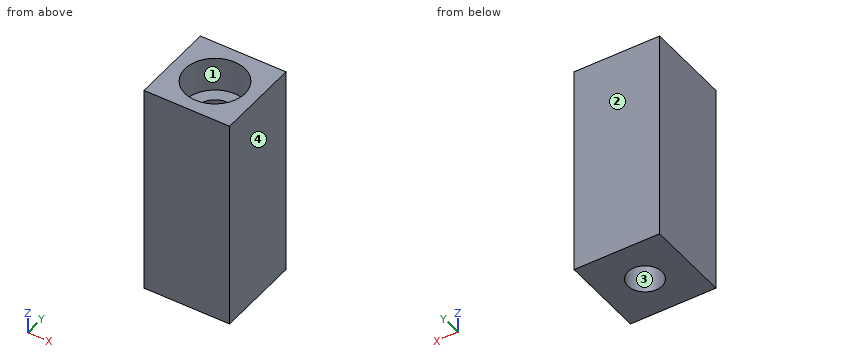
Autodesk Inventor part; units mm, degrees
ref_plane "YZ Plane" through (0, 0, 0) normal (1, 0, 0) x (0, 1, 0)
ref_plane "XZ Plane" through (0, 0, 0) normal (0, 1, 0) x (-1, 0, 0)
ref_plane "XY Plane" through (0, 0, 0) normal (0, 0, 1) x (1, 0, 0)
sketch "Sketch1" plane through (0, 0, 0) normal (0, 0, 1) x (1, 0, 0)
  line L0 (-5, -5) -> (5, -5)
  line L1 (5, -5) -> (5, 5)
  line L2 (5, 5) -> (-5, 5)
  line L3 (-5, 5) -> (-5, -5)
  line L4 (-5, -5) -> (5, 5) construction
  line L5 (5, -5) -> (-5, 5) construction
  point P0 (0, 0)
  dimension "length" = 10
  dimension "d1" = 10
extrude "Extrusion1" add sketch "Sketch1" along normal blind 25
sketch "Sketch2" plane through (0, 0, 25) normal (0, 0, 1) x (1, 0, 0)
  circle A0 centre (0, 0) radius 3.5
  dimension "diameter" = 7
extrude "Extrusion2" cut sketch "Sketch2" against normal blind 4
sketch "Sketch3" plane through (0, 0, 21) normal (0, 0, 1) x (1, 0, 0)
  circle A0 centre (0, 0) radius 2
  dimension "d9" = 4
extrude "Extrusion3" cut sketch "Sketch3" against normal blind 21
thread "Thread3"
equation "\"d1\" = length"
equation "\"d14\" = length"
properties part number "m4x0.7 25mm long"
For this review, take the finished solid that the model builds, in its own axes (mm). Face numbers are marked on the shaded views. Give positions to 0.01 mm unless a question says otherwise; leave off trailing zeros. Write each loop counter-clockwise with the first axis right and the second up, starting at its lowest first coordinate (ties: lowest second). Pieces come first, ordered by that corner, then holes. Notation, with made-up numbers: M 86,86.25 L 91,86.25 A18 cw 91,115.25 Z; hole C -31,15.5 d8. An arc over 180 degrees is marked long. One line per item, written item: value.
1) Take a section at C-C, the plane z = 8.25. Write out the cut boundary in (x, y).
Results are:
outline: M -5,-5 L 5,-5 L 5,5 L -5,5 Z; hole C 0,0 d4
2) Take a section at A-A, the plane y = 0. Write out the cut boundary in (x, z).
Results are:
outline: M -5,0 L -2,0 L -2,21 L -3.5,21 L -3.5,25 L -5,25 Z; M 2,0 L 5,0 L 5,25 L 3.5,25 L 3.5,21 L 2,21 Z
3) Take a section at D-D, the plane y = 2.5. Write out the cut boundary in (x, z), then the cut area to 3 significant figures.
Results are:
outline: M -5,0 L 5,0 L 5,25 L 2.45,25 L 2.45,21 L -2.45,21 L -2.45,25 L -5,25 Z
area: 230 mm²
4) The part is to be moulded in two halves that separate along X. For the marked faces 1, 2, 3 and 4, say which applies: +X half, -X half, draft (parallel to the pull), parting line (faces both ways), or undercut.
Results are:
face 1: undercut
face 2: draft
face 3: undercut
face 4: +X half
5) For P1, Ø5, axis at x = 1, y = -2.5, coming from the +Z side; P2, Ø4.5, axis at x = 0, y = 0, coming from the +Z side, all flat-tipped, find the tip position at first contact; note any pin that passes through.
Results are:
P1: stops at z = 25
P2: stops at z = 21
6) For line 1 (Y direction, x = 0, z = 8); line 2 (Y direction, x = 0, z = 24); line 3 (X direction, y = 3, z = 23.75), list the stretches that pass through material, from the lowest coordinate up. Write a range as from..to.
Results are:
line 1: y = -5..-2, 2..5
line 2: y = -5..-3.5, 3.5..5
line 3: x = -5..-1.8, 1.8..5
